Autodesk Inventor part; units mm, degrees
ref_plane "YZ Plane" through (0, 0, 0) normal (1, 0, 0) x (0, 1, 0)
ref_plane "XZ Plane" through (0, 0, 0) normal (0, 1, 0) x (-1, 0, 0)
ref_plane "XY Plane" through (0, 0, 0) normal (0, 0, 1) x (1, 0, 0)
sketch "Sketch1" plane through (0, 0, 0) normal (0, 0, 1) x (1, 0, 0)
  line L0 (-19, 19) -> (19, 19)
  line L1 (19, 19) -> (19, -19)
  line L2 (19, -19) -> (-19, -19)
  line L3 (-19, -19) -> (-19, 19)
  point P0 (0, 0)
  point P1 (0, 19)
  point P2 (-19, 0)
  dimension "d0" = 38
  dimension "d1" = 38
extrude "Extrusion1" add sketch "Sketch1" along normal blind 1.6
sketch "Sketch2" plane through (0, 0, 1.6) normal (0, 0, 1) x (1, 0, 0)
  circle A0 centre (-17.006, 17.006) radius 1
  line L0 (19, 19) -> (-19, 19)
  line L1 (-19, 19) -> (-19, -19)
  line L2 (19, -19) -> (19, 19)
  line L3 (-19, -19) -> (19, -19)
  ellipse E0 centre (-13.876, 13.876) end of major axis (-12.9744, 12.9744) minor radius 1.1035
  line L4 (-19, 19) -> (19, -19)
  line L5 (0, 19) -> (0, -19)
  ellipse E1 centre (13.876, 13.876) end of major axis (12.9744, 12.9744) minor radius 1.1035
  line L6 (-19, 0) -> (19, 0)
  ellipse E2 centre (-13.876, -13.876) end of major axis (-12.9744, -12.9744) minor radius 1.1035
  ellipse E3 centre (13.876, -13.876) end of major axis (12.9744, -12.9744) minor radius 1.1035
  circle A1 centre (17.006, 17.006) radius 1
  circle A2 centre (-17.006, -17.006) radius 1
  circle A3 centre (17.006, -17.006) radius 1
  point P0 (0, 0)
  dimension "d52" = 1.1035
  dimension "d53" = 1.275
  dimension "d4" = 2
  dimension "d54" = 13.876
  dimension "d60" = 13.876
  dimension "d61" = 17.006
  dimension "d62" = 17.006
extrude "Extrusion3" cut sketch "Sketch2" against normal blind 1.6 contours A0 L4 | L4 A0 | L4 E0 | E0 L4 | E3 L4 | L4 E3 | A3 L4 | L4 A3 | E1 | E2 | A1 | A2
properties part number "PCB_Camera"
Geometry check sheet. Reference: the model listing, model coordinates, mm. Coordinates: 2 decimals unless noted, no trailing zeros. One line per question, with ' | ' between items. Start each with the question number.
Item 1: Gauge pin test, flat end, axial feed: pin 1 (1.2 mm diameter, centred on x = 17.006, y = 17.006, fed in from -Z). Record the tip position at first contact, or that the pin passes through.
Item 2: Draft check along Y on faces 1 (the cylindrical face through (16.9, 18, 0.8)), 2 (the cylindrical face through (-16.47, -16.16, 0.81)), 3 (the flat face through (-19, 0, 1)), 4 (the flat face through (0, -19, 1)). Enter one of: pulls with the +Y half, pulls with the -Y half, needs draft (parallel to the pull), parting line crosses it, or undercut.
Item 3: Material ranges on L1, parallel to X at y = 13, z = 0.15; L2, parallel to Y at x = 13.5, z = 1.15, recorded low to high. Write a range as [from, to].
Item 4: Cross-section at A-A on z = 1.15. State how many separate pieces and enclosed holes the cut face has, then the cut area to 3 significant figures.
Findings:
1) pin 1: passes through
2) face 1: undercut | face 2: undercut | face 3: needs draft | face 4: pulls with the -Y half
3) L1: x = [-19, -14.55], [-12.95, 12.95], [14.55, 19] | L2: y = [-19, -14.94], [-12.7, 12.7], [14.94, 19]
4) separate pieces: 1 | enclosed holes: 8 | area: 1,410 mm²
